For this review, take the finished solid that the model builds, in its own axes (mm). A direction names the side the tool comes from. Round coordinates to 2 decimals unless told otherwise and drop trailing zeros. Write each loop counter-clockwise with the first axis right and the second up, starting at its lowest first coordinate (ties: lowest second). Pieces come first, ordered by that corner, then holes. Notation, with made-up numbers: (27.5, 4.5) - (48.5, 4.5) arc R22 cw to (48.5, 10.5) - close; hole circle Ø2 at (15.25, -9). An arc over 180 degrees is marked (long way). One line per item, written item: value. Start each with the question number.
Q1. Add section D-D on z = 0. Write out the cut boundary in (x, y).
Q2. For probe 1 along X at (y, z) = (3.75, 21); probe 2 along X at (y, z) = (3.4, -18.3); probe 3 along X at (y, z) = (8, 23), list the stretches that pass through material, from the lowest coordinate up.
Q3. Add section B-B on x = -5.5. Write out the cut boundary in (y, z).
Q4. Mouldability with a two-part tool opening along X and no side actions: class faces 1 (the face through (-8.785, 5.07, 25.465)), 2 (the face through (18, 6, 22)), 3 (the face through (20.75, 1, 9)), 4 (the face through (8.631, 2.465, -18.837)) as +X half, -X half, draft (parallel to the pull), parting line (faces both ways), or undercut.
Q5. Clearance check with flat-ended pins moving along their axes: pin 1 Ø2.5 at (x, z) = (15.5, 9.5) entering from +Y; pin 2 Ø6 at (x, y) = (12.5, 3) entering from +Z; pin 3 Ø3 at (x, z) = (16.5, 19) entering from +Y. State where each tip first meets the part, or that it passes through.
Q6. Add section A-A on y = 6.75. Write out the cut boundary in (x, z).
Q7. Add section C-C on z = -15. Write out the cut boundary in (x, y), and give its area (3 significant figures).
Q8. Tool access review of faces 5 (the face through (18.75, -1, 13)), 6 (the face through (15.276, 4.479, 22.352)), 7 (the face through (18.14, 0.47, 22.61)): name each direction out of +Z, -Z, +X, -X, +Y, -Y from which nothing blocks a thin tool from reaching the whole face with its end or side.
Autodesk Inventor part; units mm, degrees
ref_plane "Arbeitsebene1" through (0, 4, 0) normal (0, 1, 0) x (1, 0, 0)
ref_plane "YZ Plane" through (0, 0, 0) normal (1, 0, 0) x (0, 1, 0)
ref_plane "XZ Plane" through (0, 0, 0) normal (0, 1, 0) x (-1, 0, 0)
sketch "Skizze1" plane through (0, 0, 0) normal (0, 1, 0) x (-1, 0, 0)
  line L0 (-5.25, 27.5) -> (5.25, 27.5)
  line L1 (10.75, 22) -> (10.75, -22)
  line L2 (5.25, -27.5) -> (-5.25, -27.5)
  line L3 (-10.75, -22) -> (-10.75, 22)
  line L4 (-10.75, 27.5) -> (10.75, -27.5) construction
  line L5 (10.75, 27.5) -> (-10.75, -27.5) construction
  line L6 (10.75, 22) -> (5.25, 27.5)
  line L7 (10.75, -22) -> (5.25, -27.5)
  line L8 (-5.25, -27.5) -> (-10.75, -22)
  line L9 (-10.75, 22) -> (-5.25, 27.5)
  line L10 (7.25, 29.5) -> (-7.25, 29.5)
  line L11 (-12.75, 24) -> (-12.75, -24)
  line L12 (-7.25, -29.5) -> (7.25, -29.5)
  line L13 (12.75, -24) -> (12.75, 24)
  line L14 (12.75, 29.5) -> (-12.75, -29.5) construction
  line L15 (-12.75, 29.5) -> (12.75, -29.5) construction
  line L16 (12.75, 24) -> (7.25, 29.5)
  line L17 (12.75, -24) -> (7.25, -29.5)
  line L18 (-7.25, -29.5) -> (-12.75, -24)
  line L19 (-12.75, 24) -> (-7.25, 29.5)
  point P0 (0, 0)
  dimension "d0" = 21.5
  dimension "d1" = 55
  dimension "d2" = 5.5
  dimension "d3" = 5.5
  dimension "d4" = 5.5
  dimension "d5" = 5.5
  dimension "d6" = 5.5
  dimension "d7" = 5.5
  dimension "d8" = 5.5
  dimension "d9" = 5.5
  dimension "d10" = 2
  dimension "d11" = 2
  dimension "d12" = 5.5
  dimension "d13" = 5.5
  dimension "d14" = 5.5
  dimension "d15" = 5.5
  dimension "d16" = 5.5
  dimension "d17" = 5.5
  dimension "d18" = 5.5
  dimension "d19" = 5.5
extrude "Extrusion1" add sketch "Skizze1" along normal blind 10
sketch "Skizze3" plane through (0, 0, 0) normal (0, -1, 0) x (1, 0, 0)
  line L0 (7.25, -29.5) -> (-7.25, -29.5)
  line L1 (12.75, -24) -> (7.25, -29.5)
  line L2 (12.75, 24) -> (12.75, -24)
  line L3 (7.25, 29.5) -> (12.75, 24)
  line L4 (-7.25, 29.5) -> (7.25, 29.5)
  line L5 (-12.75, 24) -> (-7.25, 29.5)
  line L6 (-12.75, -24) -> (-12.75, 24)
  line L7 (-7.25, -29.5) -> (-12.75, -24)
  line L8 (-5.25, 27.5) -> (-10.75, 22)
  line L9 (5.25, 27.5) -> (-5.25, 27.5)
  line L10 (10.75, 22) -> (5.25, 27.5)
  line L11 (10.75, -22) -> (10.75, 22)
  line L12 (5.25, -27.5) -> (10.75, -22)
  line L13 (-5.25, -27.5) -> (5.25, -27.5)
  line L14 (-10.75, -22) -> (-5.25, -27.5)
  line L15 (-10.75, 22) -> (-10.75, -22)
  point P0 (0, 0)
extrude "Extrusion2" add sketch "Skizze3" along normal blind 2 contours L0 L7 L6 L5 L4 L3 L2 L1 | L9 L10 L11 L12 L13 L14 L15 L8
sketch "Skizze4" plane through (0, 0, 0) normal (0, 1, 0) x (1, 0, 0)
  line L0 (-10.75, -22) -> (-10.75, 22)
  line L1 (-10.75, -21) -> (-8.75, -21)
  line L2 (10.75, 22) -> (10.75, -22)
  line L3 (10.75, 18.3) -> (8.75, 18.3)
  circle A0 centre (-8.75, -21) radius 2
  circle A1 centre (8.75, 18.3) radius 2
  circle A2 centre (-8.75, -21) radius 0.55
  circle A3 centre (8.75, 18.3) radius 0.55
  point P0 (0, 0)
  dimension "d24" = 2
  dimension "d25" = 21
  dimension "d26" = 2
  dimension "d27" = 18.3
  dimension "d28" = 4
  dimension "d29" = 4
  dimension "d30" = 1.1
  dimension "d31" = 1.1
extrude "Extrusion3" add sketch "Skizze4" along normal blind 5
sketch "Skizze8" plane through (12.75, 10, 24) normal (1, 0, 0) x (0, 0, -1)
  line L0 (26.5, -23.1836) -> (21.5, -23.1836)
  line L1 (21.5, -23.1836) -> (21.5, 3.1836)
  line L2 (21.5, 3.1836) -> (26.5, 3.1836)
  line L3 (26.5, 3.1836) -> (26.5, -23.1836)
  line L4 (26.5, -23.1836) -> (21.5, 3.1836) construction
  line L5 (21.5, -23.1836) -> (26.5, 3.1836) construction
  point P0 (24, -10)
  dimension "d44" = 5
extrude "Extrusion7" cut sketch "Skizze8" against normal blind 8
sketch "Skizze9" plane through (0, -2, 0) normal (0, -1, 0) x (1, 0, 0)
  line L0 (4.75, -2.5) -> (4.75, 2.5)
  circle A0 centre (4.75, 0) radius 2.5
  point P0 (0, 0)
  point P1 (4.75, 2.5)
extrude "Extrusion8" cut sketch "Skizze9" against normal blind 12 contours A0 L0 picked at (4.3627, -0.7379)
sketch "Skizze17" plane through (0, 10, 0) normal (0, 1, 0) x (1, 0, 0)
  line L0 (6.25, -28) -> (-6.25, -28)
  line L1 (-11.25, -23) -> (-11.25, 23)
  line L2 (-6.25, 28) -> (6.25, 28)
  line L3 (11.25, 23) -> (11.25, -23)
  line L4 (11.25, -28) -> (-11.25, 28) construction
  line L5 (-11.25, -28) -> (11.25, 28) construction
  line L6 (-10.75, -22) -> (-10.75, 22)
  line L7 (5.25, -27.5) -> (-5.25, -27.5)
  line L8 (-11.25, -23) -> (-6.25, -28)
  line L9 (-11.25, 23) -> (-6.25, 28)
  line L10 (6.25, 28) -> (11.25, 23)
  line L11 (11.25, -23) -> (6.25, -28)
  line L12 (-5.25, -27.5) -> (-10.75, -22)
  line L13 (-10.75, 22) -> (-5.25, 27.5)
  line L14 (-5.25, 27.5) -> (5.25, 27.5)
  line L15 (5.25, 27.5) -> (10.75, 22)
  line L16 (10.75, 22) -> (10.75, 2.5)
  line L17 (10.75, -2.5) -> (10.75, -22)
  line L18 (10.75, -22) -> (5.25, -27.5)
  line L19 (12.75, -2.5) -> (10.75, -2.5)
  line L20 (10.75, -2.5) -> (10.75, 2.5)
  point P0 (0, 0)
  dimension "d74" = 0.5
  dimension "d75" = 0.5
  dimension "d80" = 5
  dimension "d81" = 5
  dimension "d82" = 5
  dimension "d83" = 5
  dimension "d84" = 5
  dimension "d85" = 5
  dimension "d86" = 5
  dimension "d87" = 5
extrude "Extrusion15" cut sketch "Skizze17" against normal up to surface (10 mm away)
sketch "Skizze18" plane through (12.75, -2, 24) normal (1, 0, 0) x (0, 0, -1)
  line L0 (21.5, 0) -> (21.5, 12)
  line L1 (0, 12) -> (21.5, 12)
  line L2 (0, 0) -> (0, 12)
  line L3 (21.5, 0) -> (0, 0)
  point P0 (24, 2)
extrude "Extrusion16" add sketch "Skizze18" along normal blind 10
ref_plane "Arbeitsebene1" through (0, 4, 0) normal (0, 1, 0) x (1, 0, 0)
sketch "Skizze19" plane through (0, 4, 0) normal (0, 1, 0) x (1, 0, 0)
  line L0 (12.75, -24) -> (7.25, -29.5)
  line L1 (4.75, -2.5) -> (22.75, -2.5)
  line L2 (12.75, -24) -> (22.75, -2.5)
  line L3 (22.75, -2.5) -> (22.75, -24)
  line L4 (22.75, -2.5) -> (22.75, -24)
  line L5 (22.75, -24) -> (12.75, -2.5)
  circle A0 centre (17.75, -13.25) radius 4.25
  line L6 (22, -13.25) -> (13.5, -13.25)
  point P0 (0, 0)
  dimension "d93" = 8.5
revolve "Umdrehung1" cut sketch "Skizze19" angle 360 about axis through (22, 4, 13.25) along (-1, 0, 0) picked at (16.8466, -10.5822) picked at (14.953, -12.931) picked at (20.1235, -11.7363) contours A0 L2 L5 | L5 L6 A0 | A0 L6 L2
sketch "Skizze20" plane through (0, 10, 0) normal (0, 1, 0) x (1, 0, 0)
  line L0 (12.75, -24) -> (22.75, -24)
  line L1 (4.75, -2.5) -> (22.75, -2.5)
  line L2 (12.75, -24) -> (22.75, -2.5)
  line L3 (22.75, -2.5) -> (12.75, -2.5)
  line L4 (12.75, -24) -> (7.25, -29.5)
  line L5 (12.75, -24) -> (12.75, -2.5)
  line L6 (22.75, -2.5) -> (22.75, -24)
  point P0 (0, 0)
extrude "Extrusion17" cut sketch "Skizze20" against normal blind 7
sketch "Skizze21" plane through (22.75, -2, 24) normal (1, 0, 0) x (0, 0, -1)
  line L0 (8.25, 12.4425) -> (13.25, 12.4425)
  line L1 (13.25, 12.4425) -> (13.25, -2.4425)
  line L2 (13.25, -2.4425) -> (8.25, -2.4425)
  line L3 (8.25, -2.4425) -> (8.25, 12.4425)
  line L4 (14.8807, 5) -> (6.6193, 5)
  line L5 (8.25, 12.4425) -> (13.25, -2.4425) construction
  line L6 (13.25, 12.4425) -> (8.25, -2.4425) construction
  point P0 (24, 2)
  point P1 (10.75, 5)
  point P2 (13.25, 5)
  point P3 (8.25, 5)
  dimension "d97" = 5
extrude "Extrusion18" cut sketch "Skizze21" against normal blind 4 contours L4 L1 L2 L3
sketch "Skizze22" plane through (22.75, -2, 24) normal (1, 0, 0) x (0, 0, -1)
  line L0 (-21.5, 10) -> (21.5, 10)
  line L1 (21.5, 10) -> (21.5, 0)
  line L2 (21.5, 0) -> (-21.5, 0)
  line L3 (-21.5, 0) -> (-21.5, 10)
  line L4 (-21.5, 10) -> (21.5, 0) construction
  line L5 (21.5, 10) -> (-21.5, 0) construction
  point P0 (24, 2)
  point P1 (0, 5)
extrude "Extrusion19" cut sketch "Skizze22" against normal blind 2
sketch "Skizze23" plane through (0, 3, 0) normal (0, 1, 0) x (1, 0, 0)
  line L0 (20.75, -15.75) -> (20.75, -24)
  line L1 (12.75, -24) -> (12.75, -2.5)
  line L2 (20.75, -21) -> (16.75, -21)
  line L3 (16.75, -21) -> (16.75, -24)
  line L4 (12.75, -24) -> (20.75, -24)
  line L5 (20.75, -5.4005) -> (16.75, -5.4005)
  line L6 (16.75, -5.4005) -> (16.75, -2.4005)
  circle A0 centre (16.75, -21) radius 1.05
  circle A1 centre (16.75, -5.4005) radius 1.05
  point P0 (0, 0)
  dimension "d102" = 4
  dimension "d103" = 3
  dimension "d104" = 4
  dimension "d105" = 3
  dimension "d106" = 2.1
  dimension "d107" = 2.1
extrude "Extrusion20" cut sketch "Skizze23" against normal through all contours A0 L3 L2 | L2 L3 A0 | A1 L6 L5 | L5 L6 A1
sketch "Skizze24" plane through (0, 3, 0) normal (0, 1, 0) x (1, 0, 0)
  point P0 (0, 0)
sketch "Skizze25" plane through (0, 3, 0) normal (0, 1, 0) x (1, 0, 0)
  circle A0 centre (16.75, -5.4005) radius 1.05
  circle A1 centre (16.75, -5.4005) radius 2
  circle A2 centre (16.75, -21) radius 1.05
  circle A3 centre (16.75, -21) radius 2
  point P0 (0, 0)
  dimension "d110" = 4
  dimension "d111" = 4
extrude "Extrusion21" add sketch "Skizze25" along normal blind 3
sketch "Skizze26" plane through (0, 3, 0) normal (0, 1, 0) x (1, 0, 0)
  point P0 (0, 0)
chamfer "Fase2" distance 4 angle 45 2 edges at (20.75, 0.5, 2.5) (20.75, 0.5, 24)
fillet "Rundung2" radius 4 2 edges at (20.75, 0.5, 20) (20.75, 0.5, 6.5)
equation "\"d3\" = d2"
equation "\"d5\" = d4"
equation "\"d6\" = d4"
equation "\"d7\" = d6"
equation "\"d8\" = d4"
equation "\"d9\" = d8"
equation "\"d13\" = d12"
equation "\"d14\" = d12"
equation "\"d15\" = d14"
equation "\"d16\" = d12"
equation "\"d17\" = d16"
equation "\"d18\" = d12"
equation "\"d19\" = d18"
equation "\"d83\" = d82"
equation "\"d84\" = d82"
equation "\"d85\" = d84"
equation "\"d86\" = d82"
equation "\"d87\" = d86"
properties part number "CameraMold"
Result set:
1. outline: (-12.75, -2) - (2.25, -2) - (2.25, 0) - (-11.25, 0) - (-11.25, 10) - (-12.75, 10) - close
2. probe 1: x = -12.75 to -11.25, -10.75 to -9.3, -8.2 to -6.75, 11.25 to 12.75, 14.75 to 15.7, 17.8 to 18.75
2. probe 2: x = -12.75 to -11.25, 6.75 to 8.2, 9.3 to 10.75, 11.25 to 12.75
2. probe 3: x = -12.75 to -11.25, 11.25 to 12.75
3. outline: (-2, -29.5) - (10, -29.5) - (10, -28) - (0, -28) - (0, 28) - (10, 28) - (10, 29.5) - (-2, 29.5) - close
4. face 1: undercut
4. face 2: draft
4. face 3: +X half
4. face 4: undercut
5. pin 1: stops at y = 3
5. pin 2: stops at z = 27.25
5. pin 3: stops at y = 6
6. outline: (-12.75, -24) - (-7.25, -29.5) - (7.25, -29.5) - (12.75, -24) - (12.75, -2.5) - (11.25, -2.5) - (11.25, -23) - (6.25, -28) - (-6.25, -28) - (-11.25, -23) - (-11.25, 23) - (-6.25, 28) - (6.25, 28) - (11.25, 23) - (11.25, 2.5) - (12.75, 2.5) - (12.75, 24) - (7.25, 29.5) - (-7.25, 29.5) - (-12.75, 24) - close
7. outline: (-12.75, -2) - (12.75, -2) - (12.75, 10) - (11.25, 10) - (11.25, 0) - (-11.25, 0) - (-11.25, 10) - (-12.75, 10) - close
7. area: 81.0 mm^2
8. face 5: +X, +Y, -Y
8. face 6: +Y
8. face 7: +Z, +X, +Y, -Y
